For this review, take the finished solid that the model builds, in its own axes (mm). Face numbers are marked on the shaded views. A direction names the side the tool comes from. Round coordinates to 2 decimals unless told otherwise and drop trailing zeros. Order: outer loops, then holes, each group sorted by start corner. A loop starts at its lowest first (then second) coordinate and runs counter-clockwise, first axis right, second up. Notation, with made-up numbers: (36, 40) -> (56, 40) arc R17 ccw to (56, 62) -> close; hole circle Ø1 at (69, 1). An arc over 180 degrees is marked (long way). Put each result on its own line as item: value. Start each with the question number.
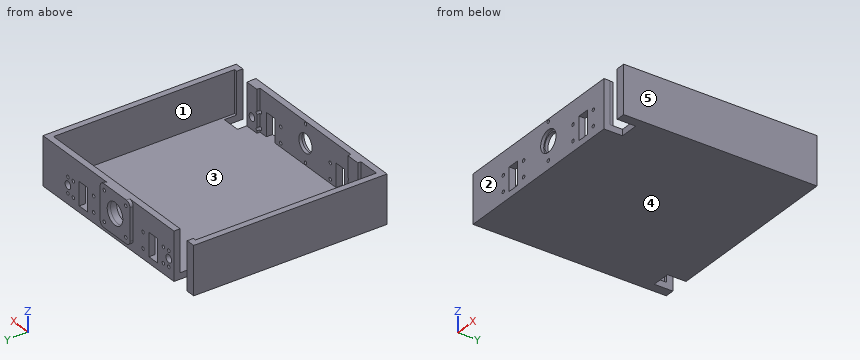
```python
from build123d import *

# Parameters (mm, degrees)
F0_W      = 217.3440154
F0_H      = 198.6000092
F1_DEPTH  = 6.35
F2_W      = 217.3440154
F2_H      = 198.6000092
F2_W_2    = 204.6440154
F2_H_2    = 185.9000092
F3_DEPTH  = 43.0059846
F4_R      = 1.7272
F4_R_2    = 11.2530001
F4_R_3    = 4
F5_DEPTH  = 6.35
F6_DEPTH  = 6.35
F7_R      = 11.1125
F8_DEPTH  = 3.175
F9_R      = 9.525
F10_DEPTH = 3.175
F11_R     = 1.7272
F12_DEPTH = 6.35
F14_DEPTH = 3.175
F15_DEPTH = 3.175
F16_R     = 1.7272
F17_DEPTH = 6.35
F18_W     = 12.2546872
F18_H     = 24
F18_R     = 1.7272
F19_DEPTH = 198.6000092
F20_R     = 3.175
F21_DEPTH = 4.7625
F22_W     = 43.0059846
F22_H     = 43.0059846
F22_R     = 1.7272
F22_R_2   = 11.2530001
F23_DEPTH = 3.41249
F24_R     = 5.08
F25_W     = 19.05
F25_H     = 19.05
F26_DEPTH = 49.3559846


# Not quite as in the source:
# - a feature names something its author has since deleted; it is built from what else it names


with BuildPart() as f1:
    # F0 (on Top) → F1 (new body)
    with BuildSketch(Plane.XY):
        with Locations((108.6720077, -99.3000046)):
            Rectangle(F0_W, F0_H)
    extrude(amount=F1_DEPTH)

    # F2 (on face) → F3 (join)
    with BuildSketch(Plane.XY.offset(6.35)):
        with Locations((108.6720077, -99.3000046)):
            Rectangle(F2_W, F2_H)
        with Locations((108.6720077, -99.3000046)):
            Rectangle(F2_W_2, F2_H_2, mode=Mode.SUBTRACT)
    extrude(amount=F3_DEPTH)

    # F4 (on face) → F5 (cut, through all)
    with BuildSketch(Plane(origin=(0, 0, 0), x_dir=(-1, 0, 0), z_dir=(0, 1, 0))):
        with Locations((-124.1720021, 43.3529867)):
            Circle(F4_R)
        with Locations((-93.1720133, 43.3529867)):
            Circle(F4_R)
        with Locations((-124.1720021, 12.3529979)):
            Circle(F4_R)
        with Locations((-108.6720077, 27.8529923)):
            Circle(F4_R_2)
        with Locations((-93.1720133, 12.3529979)):
            Circle(F4_R)
        with Locations((-181.4220019, 18.6124977)):
            Circle(F4_R_3)
        with Locations((-35.9220135, 18.6124977)):
            Circle(F4_R_3)
    extrude(amount=-F5_DEPTH, mode=Mode.SUBTRACT)

    # F4 (on face) → F6 (cut, through all)
    with BuildSketch(Plane(origin=(0, 0, 0), x_dir=(-1, 0, 0), z_dir=(0, 1, 0))):
        with Locations((-124.1720021, 43.3529867)):
            Circle(F4_R)
        with Locations((-93.1720133, 43.3529867)):
            Circle(F4_R)
        with Locations((-124.1720021, 12.3529979)):
            Circle(F4_R)
        with Locations((-108.6720077, 27.8529923)):
            Circle(F4_R_2)
        with Locations((-93.1720133, 12.3529979)):
            Circle(F4_R)
        with Locations((-181.4220019, 18.6124977)):
            Circle(F4_R_3)
        with Locations((-35.9220135, 18.6124977)):
            Circle(F4_R_3)
    extrude(amount=-F6_DEPTH, mode=Mode.SUBTRACT)

    # F7 (on face) → F8 (cut)
    with BuildSketch(Plane.XZ.offset(198.6000092)):
        with Locations((108.6720077, 27.8529923)):
            Circle(F7_R)
    extrude(amount=-F8_DEPTH, mode=Mode.SUBTRACT)

    # F9 (on face) → F10 (cut, through all)
    with BuildSketch(Plane.XZ.offset(195.4250092)):
        with Locations((108.6720077, 27.8529923)):
            Circle(F9_R)
    extrude(amount=-F10_DEPTH, mode=Mode.SUBTRACT)

    # F11 (on face) → F12 (cut, through all)
    with BuildSketch(Plane.XZ.offset(198.6000092)):
        with Locations((108.6720077, 46.9029923)):
            Circle(F11_R)
        with Locations((108.6720077, 8.8029923)):
            Circle(F11_R)
    extrude(amount=-F12_DEPTH, mode=Mode.SUBTRACT)

    # F13 (on face) → F14 (join)
    with BuildSketch(Plane(origin=(0, -192.2500092, 0), x_dir=(-1, 0, 0), z_dir=(0, 1, 0))):
        Polygon((-28.7470088, 6.35), (-28.7470088, 49.3559846), (-35.9220135, 49.3559846), (-43.0970182, 49.3559846), (-43.0970182, 6.35), align=None)
        with BuildLine():
            ThreePointArc((-31.9220135, 18.6124977), (-38.7504406247, 15.7840705753), (-35.9220135, 22.6124977))
            ThreePointArc((-35.9220135, 22.6124977), (-33.0935863753, 21.4409248247), (-31.9220135, 18.6124977))
        make_face(mode=Mode.SUBTRACT)
        Polygon((-174.2469972, 6.35), (-174.2469972, 49.3559846), (-181.4220019, 49.3559846), (-188.5970066, 49.3559846), (-188.5970066, 6.35), align=None)
        with BuildLine():
            ThreePointArc((-177.4220019, 18.6124977), (-184.2504290247, 15.7840705753), (-181.4220019, 22.6124977))
            ThreePointArc((-181.4220019, 22.6124977), (-178.5935747753, 21.4409248247), (-177.4220019, 18.6124977))
        make_face(mode=Mode.SUBTRACT)
    extrude(amount=F14_DEPTH)

    # F15 (cut): faces of the model
    f15_faces = [f1.faces().sort_by_distance(p)[0] for p in [
        (181.4220019, -192.2500092, 18.6124977),
        (35.9220135, -192.2500092, 18.6124977),
    ]]
    extrude(f15_faces, amount=-F15_DEPTH, mode=Mode.SUBTRACT)

    # F16 (on face) → F17 (cut, through all)
    with BuildSketch(Plane(origin=(0, 0, 0), x_dir=(-1, 0, 0), z_dir=(0, 1, 0))):
        with Locations((-181.4220019, 10.6437477)):
            Circle(F16_R)
        with Locations((-181.4220019, 26.5812477)):
            Circle(F16_R)
        with Locations((-35.9220135, 10.6437477)):
            Circle(F16_R)
        with Locations((-35.9220135, 26.5812477)):
            Circle(F16_R)
    extrude(amount=-F17_DEPTH, mode=Mode.SUBTRACT)

    # F18 (on face) → F19 (cut, through all)
    with BuildSketch(Plane.XZ.offset(198.6000092)):
        with Locations((158.9532508, 18.35)):
            Rectangle(F18_W, F18_H)
        with Locations((173.5969985, 26.3812514)):
            Circle(F18_R)
        with Locations((173.5969985, 10.3187486)):
            Circle(F18_R)
        with Locations((144.3095031, 26.3812514)):
            Circle(F18_R)
        with Locations((144.3095031, 10.3187486)):
            Circle(F18_R)
        with Locations((58.3907646, 18.35)):
            Rectangle(F18_W, F18_H)
        with Locations((43.7470169, 26.3812514)):
            Circle(F18_R)
        with Locations((73.0345123, 26.3812514)):
            Circle(F18_R)
        with Locations((73.0345123, 10.3187486)):
            Circle(F18_R)
        with Locations((43.7470169, 10.3187486)):
            Circle(F18_R)
    extrude(amount=-F19_DEPTH, mode=Mode.SUBTRACT)

    # F20 (on face) → F21 (cut)
    with BuildSketch(Plane.XZ.offset(6.35)):
        with Locations((93.1720133, 43.3529867)):
            Circle(F20_R)
        with Locations((124.1720021, 43.3529867)):
            Circle(F20_R)
        with Locations((124.1720021, 12.3529979)):
            Circle(F20_R)
        with Locations((93.1720133, 12.3529979)):
            Circle(F20_R)
    extrude(amount=-F21_DEPTH, mode=Mode.SUBTRACT)

    # F22 (on face) → F23 (join)
    with BuildSketch(Plane(origin=(0, 0, 0), x_dir=(-1, 0, 0), z_dir=(0, 1, 0))):
        with Locations((-108.6720077, 27.8529923)):
            Rectangle(F22_W, F22_H)
        with Locations((-124.1720021, 12.3529979)):
            Circle(F22_R, mode=Mode.SUBTRACT)
        with Locations((-93.1720133, 12.3529979)):
            Circle(F22_R, mode=Mode.SUBTRACT)
        with Locations((-124.1720021, 43.3529867)):
            Circle(F22_R, mode=Mode.SUBTRACT)
        with Locations((-108.6720077, 27.8529923)):
            Circle(F22_R_2, mode=Mode.SUBTRACT)
        with Locations((-93.1720133, 43.3529867)):
            Circle(F22_R, mode=Mode.SUBTRACT)
    extrude(amount=F23_DEPTH)

    # F24
    f24_edges = [f1.edges().sort_by_distance(p)[0] for p in [
        (87.169015, 1.706245, 49.355985),
        (130.175, 1.706245, 49.355985),
        (87.169015, 1.706245, 6.35),
        (130.175, 1.706245, 6.35),
    ]]
    fillet(f24_edges, radius=F24_R)

    # F25 (on face) → F26 (cut, through all)
    with BuildSketch(Plane(origin=(0, 0, 0), x_dir=(1, 0, 0), z_dir=(0, 0, -1))):
        with Locations((198.4470123, 189.0750092)):
            Rectangle(F25_W, F25_H)
        with Locations((18.8970031, 9.525)):
            Rectangle(F25_W, F25_H)
    extrude(amount=-F26_DEPTH, mode=Mode.SUBTRACT)


solid = f1.part
```
Item 1: Consider section B-B, the plane x = 200. Write out the cut boundary in (y, z), plus the area to 3 significant figures.
Item 2: For L1, parallel to Y at x = 33, z = 26 (3 decimals); L2, parallel to X at y = -112.5, z = 29.5; L3, parallel to Y at x = 144.5, z = 18, list the stretches that pass through material, from the lowest coordinate up.
Item 3: Insertion check: pin 1 Ø7 at (x, z) = (23.5, 4) entering from +Y; pin 2 Ø2 at (x, y) = (169.5, -151) entering from -Z; pin 3 Ø3 at (x, z) = (43.75, 10.32) entering from -Y; pin 4 Ø2 at (x, z) = (93.17, 43.35) entering from +Y. Each pin has a flat end and moves straight along its axis. Give the tip position at first contact, or say it passes through.
Item 4: Consider section C-C, the plane z = 33. Count the separate pieces of the cut face and the enclosed holes in it, plus the area to 3 significant figures.
Item 5: Tool access review of the marked faces 1 and 2: name each direction out of +Z, -Z, +X, -X, +Y, -Y from which nothing blocks a thin tool from reaching the whole face with its end or side.
Item 6: Consider section A-A, the plane y = -119.5. Write out the cut boundary in (x, z).
Item 7: Mouldability with a two-part tool opening along X and no side actions: class the marked faces 3, 4 and 5 as +X half, -X half, draft (parallel to the pull), parting line (faces both ways), or undercut.
Evaluation:
1. outline: (-179.55, 0) -> (0, 0) -> (0, 49.36) -> (-6.35, 49.36) -> (-6.35, 6.35) -> (-179.55, 6.35) -> close
1. area: 1,410 mm^2
2. L1: y = -198.6 to -189.075, -6.35 to 0
2. L2: x = 0 to 6.35, 210.99 to 217.34
2. L3: y = -198.6 to -192.25, -6.35 to 0
3. pin 1: stops at y = -19.05
3. pin 2: stops at z = 0
3. pin 3: passes through
3. pin 4: stops at y = -192.25
4. separate pieces: 4
4. enclosed holes: 0
4. area: 4,810 mm^2
5. face 1: +Z
5. face 2: +Z, -Z, +X, -X, -Y
6. outline: (0, 0) -> (217.34, 0) -> (217.34, 49.36) -> (210.99, 49.36) -> (210.99, 6.35) -> (6.35, 6.35) -> (6.35, 49.36) -> (0, 49.36) -> close
7. face 3: undercut
7. face 4: draft
7. face 5: +X half
